Input: dimensioned drawing with shaded views. Units: mm. Origin: part minimum x, y, z. Coordinates: 2 decimals unless noted, no trailing zeros. Loops run counter-clockwise (first coordinate to the right, second up) from the corner with the lowest first, then second, coordinate; pieces in that order, holes last. Notation, with made-up numbers: (23.25, 56) - (55.25, 56) arc R23 cw to (55.25, 65) - close; hole circle Ø6 at (57, 86.5). An arc over 180 degrees is marked (long way). Put each result on its own line as item: value. Start each with the question number.
1) Contact query for flat-ended pins moving along their axis: pin 1 Ø1 at (x, z) = (153.5, 1) entering from +Y; pin 2 Ø1 at (x, z) = (96.5, 2) entering from -Y; pin 3 Ø1.6 at (y, z) = (112.5, 1.5) entering from -X. Output: stop coordinate, or through.
2) Section B-B on z = 0.5. Count the separate pieces of the cut face and the enclosed holes in it, and give its area (3 significant figures).
3) Section D-D on x = 77. Output: boundary loops of the cut face in (y, z) (1 decimal).
4) Material intervals for line 1 along X through (y, z) = (25, 2.35) (1 decimal); line 2 along Y through (x, z) = (125, 2.2); line 3 along X through (y, z) = (5.5, 0.4) (1 decimal), sorted ascending. Write a range as from..to.
5) Section C-C on x = 168. Output: boundary loops of the cut face in (y, z) (1 decimal).
6) Section A-A on y = 107. Output: boundary loops of the cut face in (x, z) (1 decimal).
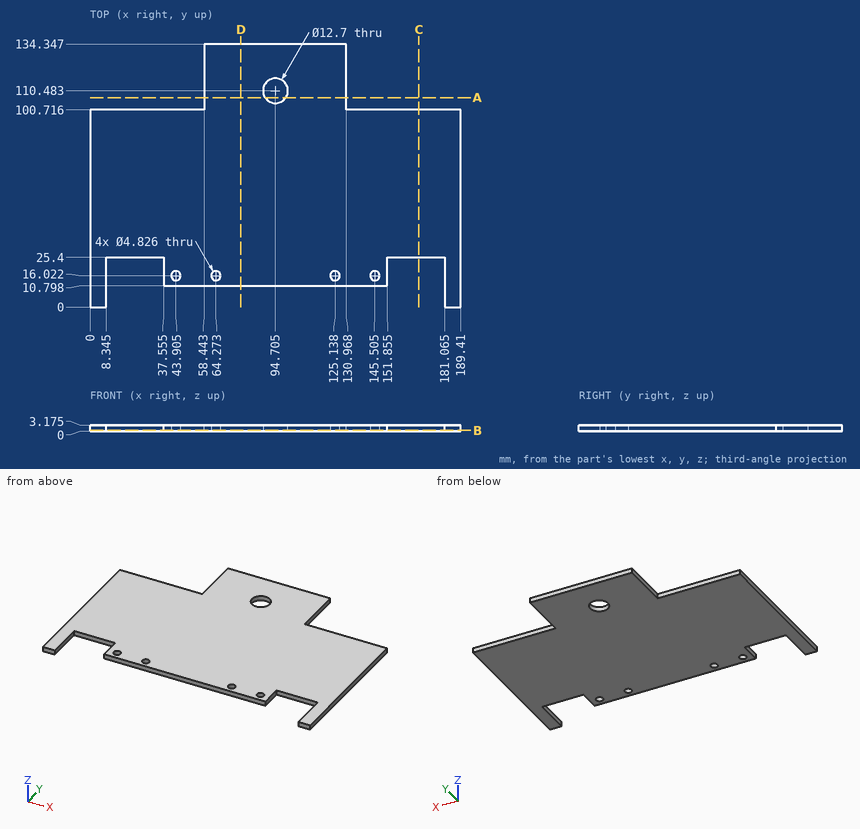
Answer block:
1. pin 1: stops at y = 100.72
1. pin 2: stops at y = 10.8
1. pin 3: stops at x = 58.44
2. separate pieces: 1
2. enclosed holes: 5
2. area: 18,600 mm²
3. outline: (10.8, 0) - (134.3, 0) - (134.3, 3.2) - (10.8, 3.2) - close
4. line 1: x = 0..8.3, 37.6..151.9, 181.1..189.4
4. line 2: y = 10.8..13.61, 18.43..134.35
4. line 3: x = 0..8.3, 181.1..189.4
5. outline: (25.4, 0) - (100.7, 0) - (100.7, 3.2) - (25.4, 3.2) - close
6. outline: (58.4, 0) - (89.4, 0) - (89.4, 3.2) - (58.4, 3.2) - close; (100, 0) - (131, 0) - (131, 3.2) - (100, 3.2) - close
